```python
from build123d import *

# Parameters (mm, degrees)
SKETCH_2_R = 4


with BuildPart() as part:
    # По траектории1: sweep along a path in Эскиз1
    with BuildLine(Plane(origin=(0, 0, 0), x_dir=(0, 0, -1), z_dir=(1, 0, 0))) as sweep_1_path:
        Line((0, -15), (35, -15))
        ThreePointArc((35, -15), (42.071067812, -12.071067812), (45, -5))
        Line((45, -5), (45, 5))
        ThreePointArc((45, 5), (42.071067812, 12.071067812), (35, 15))
        Line((35, 15), (0, 15))
    # Эскиз2 → По траектории1 (sweep)
    with BuildSketch(Plane.XY):
        with Locations((0, -15)):
            Circle(SKETCH_2_R)
    sweep(path=sweep_1_path.line)


solid = part.part
```
Work out the finished part from the listing and answer in its coordinate system (mm). A direction names the side the tool comes from. Give positions to 0.01 mm unless a question says otherwise; leave off trailing zeros. Write each loop counter-clockwise with the first axis right and the second up, starting at its lowest first coordinate (ties: lowest second). Pieces come first, ordered by that corner, then holes. Notation, with made-up numbers: (63, 60.25) - (74, 60.25) arc R17 ccw to (74, 75.25) - close; hole circle Ø3 at (19.5, 63.5). An arc over 180 degrees is marked (long way). Use one line per item in the form item = value.
1. Determine the mould class of faces 3 (the face through (0, 15, 0)), 4 (the face through (1.846, 0.07, -41.451)) for opening direction Y: released by +Y, released by -Y, zero draft, split by the parting line, or undercut.
Filled in:
face_3 = zero draft
face_4 = undercut
2. Each of these flat-tipped pins is pushed along its axis until it touches: pin 1 Ø1.5 at (x, z) = (1.5, -36) entering from -Y; pin 2 Ø2 at (x, z) = (-2.5, -23.5) entering from -Y. Where does it stop, or does it pass through?
Filled in:
pin_1 = -18.9
pin_2 = -18.71
3. A cutting plane is placed at C-C (y = -1). Write down the section's boundary in (x, z), and give its area (3 significant figures).
Filled in:
outline = circle Ø8 at (0, -45)
area = 50.3 mm^2
4. Consider L1, parallel to Y at x = -0.25, z = -12.5; L2, parallel to Y at x = 2.5, z = -31; L3, parallel to Z at x = -0.5, y = -15. Determine where each line is inside the solid, lowest interval first.
Filled in:
L1 = -18.99 to -11.01, 11.01 to 18.99
L2 = -18.12 to -11.88, 11.88 to 18.12
L3 = -44.75 to 0
5. A cutting plane is placed at A-A (x = 0). Write down the section's boundary in (y, z), and give its area (3 significant figures).
Filled in:
outline = (-19, -35) arc R14 ccw to (-5, -49) - (5, -49) arc R14 ccw to (19, -35) - (19, 0) - (11, 0) - (11, -35) arc R6 cw to (5, -41) - (-5, -41) arc R6 cw to (-11, -35) - (-11, 0) - (-19, 0) - close
area = 891 mm^2
6. A cutting plane is placed at D-D (x = -2.75). Write down the section's boundary in (y, z).
Filled in:
outline = (-17.9, -35) arc R12.9 ccw to (-5, -47.9) - (5, -47.9) arc R12.9 ccw to (17.9, -35) - (17.9, 0) - (12.1, 0) - (12.1, -35) arc R7.1 cw to (5, -42.1) - (-5, -42.1) arc R7.1 cw to (-12.1, -35) - (-12.1, 0) - (-17.9, 0) - close
7. For faces 1 (the face through (0, -15, 0)), 2 (the face through (-0.521, 18.966, -17.255)), determine the directions among +Z, -Z, +X, -X, +Y, -Y from which every point of the face is accessible in a straight line to the end or side of a thin tool.
Filled in:
face_1 = +Z, +X, -X, +Y, -Y
face_2 = +Z
8. A cutting plane is placed at B-B (z = -11.5). Write down the section's boundary in (x, y).
Filled in:
outline = circle Ø8 at (0, -15); circle Ø8 at (0, 15)
